Model file for the job. Use its own axes, mm. Coordinates: 2 decimals unless noted, no trailing zeros. Loops run counter-clockwise (first coordinate to the right, second up) from the corner with the lowest first, then second, coordinate; pieces in that order, holes last. Notation, with made-up numbers: M -25,19.5 L -2,19.5 A5 ccw -2,27.5 Z; hole C 35,19 d3. An arc over 180 degrees is marked long. Write item = value, one per line. Start each with the question number.
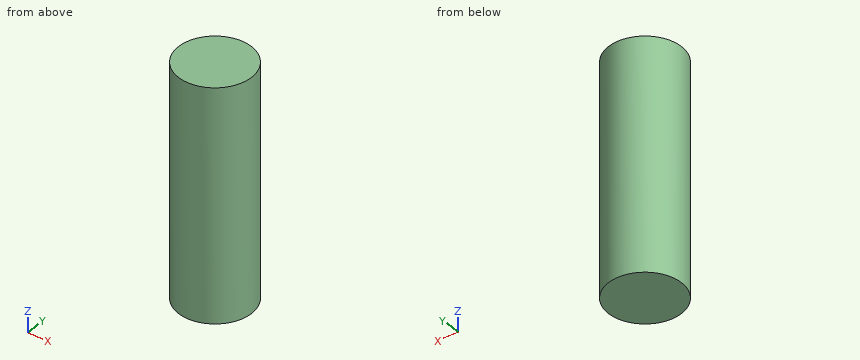
from build123d import *

# Parameters (mm, degrees)
F0_R     = 12.0559653511
F1_DEPTH = 101.6
F3_DEPTH = 76.2


with BuildPart() as f1:
    # F0 (on Top) → F1 (new body)
    with BuildSketch(Plane.XY):
        Circle(F0_R)
    extrude(amount=F1_DEPTH)


with BuildPart() as f3:
    # F0 (on Top) → F3 (new body)
    with BuildSketch(Plane.XY):
        Circle(F0_R)
    extrude(amount=F3_DEPTH)


solid = f3.part
Item 1: Probe L1, parallel to X at y = 0.25, z = 42; L2, parallel to X at y = -8.25, z = 36; L3, parallel to Y at x = 4.5, z = 38. List the from-to ranges inside material, lowest first.
Item 2: Pin check, flat tips, straight feed: pin 1 Ø10 at (x, z) = (-7, 53.5) entering from +Y; pin 2 Ø2 at (y, z) = (0.5, 12) entering from -X; pin 3 Ø8 at (x, z) = (5, 64.5) entering from -Y; pin 4 Ø12 at (x, z) = (-9, 29) entering from -Y. Stop position of each tip, or through.
Item 3: Cut at A-A (z = 54). Give the cut face in (x, y), plus the area to 3 significant figures.
Item 4: Cut at B-B (y = 6.5). Give the cut face in (x, z), plus the area to 3 significant figures.
Item 5: Cut at C-C (x = 8). Give the cut face in (y, z), plus the area to 3 significant figures.
Reported:
q1.L1 = -12.05 to 12.05
q1.L2 = -8.79 to 8.79
q1.L3 = -11.18 to 11.18
q2.pin_1 = 11.89
q2.pin_2 = -12.06
q2.pin_3 = -12.01
q2.pin_4 = -11.68
q3.outline = C 0,0 d24.11
q3.area = 457 mm^2
q4.outline = M -10.15,0 L 10.15,0 L 10.15,76.2 L -10.15,76.2 Z
q4.area = 1,550 mm^2
q5.outline = M -9.02,0 L 9.02,0 L 9.02,76.2 L -9.02,76.2 Z
q5.area = 1,370 mm^2
